Read the model definition and answer for the solid it produces. Units are mm, in the model's axes. A direction names the side the tool comes from. Round coordinates to 2 decimals unless told otherwise and drop trailing zeros. Order: outer loops, then holes, each group sorted by start corner. A loop starts at its lowest first (then second) coordinate and runs counter-clockwise, first axis right, second up. Notation, with made-up numbers: (46, -9) - (91, -9) arc R23 ccw to (91, 9) - close; hole circle Ø9 at (16, 54.5). An arc over 180 degrees is marked (long way). Put each result on its own line as item: value. Start each with the question number.
Q1. Each of these flat-tipped pins is pushed along its axis until it touches: pin 1 Ø3.5 at (x, z) = (1, 2.5) entering from +Y; pin 2 Ø2.5 at (x, z) = (12, 2) entering from -Y; pin 3 Ø3.5 at (y, z) = (4.5, 0.5) entering from +X; pin 4 Ø1.8 at (x, z) = (-12.87, 0) entering from -Y. Where does it stop, or does it pass through?
Q2. Which of the six approach directions +Z, -Z, +X, -X, +Y, -Y give full straight-line access (tool end or side, diameter ignored) to faces 4 (the face through (-10.5, 8, 0)), 5 (the face through (10.5, 21, 0)), 6 (the face through (-15, 18, -0.5)), 7 (the face through (10.5, 8, 0)), 8 (the face through (-13, 19, 1.4))?
Q3. Section C-C on y = 25.5 is taken. Give the vertices of the cut face in (x, z) (3 decimals).
Q4. Find the intervals of material crossed by line 1 along Y through (x, z) = (12, -1.5); line 2 along Y through (x, z) = (-8.5, 5); line 3 along X through (y, z) = (18.3, 0), in increasing order. Write a range as from..to.
Q5. For a pull along X with two mould halves and no side action, classify faces 1 (the face through (3, 11, 6)), 2 (the face through (3, 25, 0)), 3 (the face through (-11.872, 17.732, -0.037)) as pulls with the +X half, pulls with the -X half, needs draft (parallel to the pull), parting line crosses it, or undercut.
Q6. Section A-A on x = -3 is taken. Give the vertices of the cut face in (y, z), then the cut area to 3 significant figures.
Q7. Section B-B on z = 5 is taken. Give the vertices of the cut face in (x, y).
Q8. Section D-D on z = -3.5 is taken. Give the vertices of the cut face in (x, y).
from build123d import *

# Parameters (mm, degrees)
SKETCH1_W               = 21
SKETCH1_H               = 12
BOSS_EXTRUDE1_DEPTH     = 23
SKETCH2_W               = 5
SKETCH2_H               = 2.5
BOSS_EXTRUDE2_DEPTH     = 12
CUT_EXTRUDE2_DEPTH      = 29.376927247
CUT_EXTRUDE2_DEPTH_BACK = 12
BOSS_EXTRUDE3_DEPTH     = 4.5
SKETCH5_R               = 2.5
BOSS_EXTRUDE4_DEPTH     = 3


with BuildPart() as part:
    # Sketch1 → Boss-Extrude1 (new body)
    with BuildSketch(Plane(origin=(0, 0, 0), x_dir=(1, 0, 0), z_dir=(0, 1, 0))):
        Rectangle(SKETCH1_W, SKETCH1_H)
    extrude(amount=BOSS_EXTRUDE1_DEPTH)

    # Sketch2 → Boss-Extrude2 (add)
    with BuildSketch(Plane.XY.offset(6)):
        with Locations((13, 17.75)):
            Rectangle(SKETCH2_W, SKETCH2_H)
        with Locations((-13, 17.75)):
            Rectangle(SKETCH2_W, SKETCH2_H)
    extrude(amount=-BOSS_EXTRUDE2_DEPTH)

    # Sketch3 → Cut-Extrude2 (cut, two sides: drawn at the far end of the back side and taken through both)
    with BuildSketch(Plane(origin=(0, 23, 0), x_dir=(1, 0, 0), z_dir=(0, 1, 0)).offset(-CUT_EXTRUDE2_DEPTH_BACK)):
        with BuildLine():
            Line((15.5, 0.5), (15.5, -0.5))
            Line((15.5, -0.5), (13.737359872, -0.5))
            ThreePointArc((13.737359872, -0.5), (11.871334468, 0), (13.737359872, 0.5))
            Line((13.737359872, 0.5), (15.5, 0.5))
        make_face()
        with BuildLine():
            Line((-15.5, 0.5), (-13.737359872, 0.5))
            ThreePointArc((-13.737359872, 0.5), (-11.871334468, 0), (-13.737359872, -0.5))
            Line((-13.737359872, -0.5), (-15.5, -0.5))
            Line((-15.5, -0.5), (-15.5, 0.5))
        make_face()
    extrude(amount=CUT_EXTRUDE2_DEPTH + CUT_EXTRUDE2_DEPTH_BACK, mode=Mode.SUBTRACT)

    # Sketch4 → Boss-Extrude3 (add)
    with BuildSketch(Plane(origin=(0, 23, 0), x_dir=(1, 0, 0), z_dir=(0, 1, 0))):
        with BuildLine():
            ThreePointArc((0.975, 2.454460226), (-10.5, 0), (0.975, -2.454460226))
            ThreePointArc((0.975, -2.454460226), (3, 0), (0.975, 2.454460226))
        make_face()
    extrude(amount=BOSS_EXTRUDE3_DEPTH)

    # Sketch5 → Boss-Extrude4 (add)
    with BuildSketch(Plane(origin=(0, 27.5, 0), x_dir=(1, 0, 0), z_dir=(0, 1, 0))):
        with Locations(Location((-4.5, 0, 0), (0, 0, 270))):
            Circle(SKETCH5_R)
    extrude(amount=BOSS_EXTRUDE4_DEPTH)


solid = part.part
Findings:
1. pin 1: y = 27.5
1. pin 2: y = 16.5
1. pin 3: x = 10.5
1. pin 4: through
2. face 4: +Z, -Z, -X, -Y
2. face 5: +Z, -Z, +X, +Y
2. face 6: -X, +Y, -Y
2. face 7: +Z, -Z, +X, -Y
2. face 8: +Z, -Z, -X, +Y
3. outline: (0.975, -2.454) arc R2.5 ccw to (0.975, 2.454) arc R6 ccw (long way) to start
4. line 1: 16.5..19
4. line 2: 0..23
4. line 3: -11.87..11.87
5. face 1: needs draft
5. face 2: pulls with the +X half
5. face 3: undercut
6. outline: (0, -6) - (23, -6) - (23, -5.81) - (27.5, -5.81) - (27.5, -2) - (30.5, -2) - (30.5, 2) - (27.5, 2) - (27.5, 5.81) - (23, 5.81) - (23, 6) - (0, 6) - close
6. area: 340 mm2
7. outline: (-15.5, 16.5) - (-10.5, 16.5) - (-10.5, 0) - (10.5, 0) - (10.5, 16.5) - (15.5, 16.5) - (15.5, 19) - (10.5, 19) - (10.5, 23) - (-1.18, 23) - (-1.18, 27.5) - (-7.82, 27.5) - (-7.82, 23) - (-10.5, 23) - (-10.5, 19) - (-15.5, 19) - close
8. outline: (-15.5, 16.5) - (-10.5, 16.5) - (-10.5, 0) - (10.5, 0) - (10.5, 16.5) - (15.5, 16.5) - (15.5, 19) - (10.5, 19) - (10.5, 23) - (0.37, 23) - (0.37, 27.5) - (-9.37, 27.5) - (-9.37, 23) - (-10.5, 23) - (-10.5, 19) - (-15.5, 19) - close
